from build123d import *


with BuildPart() as part:
    # Sketch1 → Revolve1 (revolve)
    with BuildSketch(Plane.XY, mode=Mode.PRIVATE) as revolve1_sk:
        Polygon((4.8, 24), (4.8, 22), (8.8, 22), (8.8, 20), (4.8, 20.000000056), (4.8, 18), (4.8, 16), (8.8, 16), (8.8, 14), (4.8, 14), (4.8, 11), (4.8, 10), (8.8, 10), (8.8, 8), (4.8, 8), (4.8, 5), (4.8, 4), (8.8, 4), (8.8, 2), (4.8, 2), (4.8, -1), (4.8, -2), (8.8, -2), (8.8, -4), (4.8, -4), (4.8, -7), (4.8, -8), (8.8, -8), (8.8, -10), (4.8, -10), (4.8, -13), (4.8, -14), (8.8, -14), (8.8, -16), (4.8, -16), (4.8, -19), (4.8, -20), (8.8, -20), (8.8, -22), (4.8, -22), (4.8, -24), (4.8, -27), (0, -27), (0, 27), (4.8, 27), align=None)
    revolve(revolve1_sk.sketch.rotate(Axis((0, 27, 0), (0, -1, 0)), 180), axis=Axis((0, 27, 0), (0, -1, 0)))


solid = part.part
The model under review builds one solid part; all positions refer to its coordinate system, in mm. A direction names the side the tool comes from. Give positions to 0.01 mm unless a question says otherwise; leave off trailing zeros. Order: outer loops, then holes, each group sorted by start corner. A loop starts at its lowest first (then second) coordinate and runs counter-clockwise, first axis right, second up. Notation, with made-up numbers: M 82.5,8.5 L 133.5,8.5 A10 cw 133.5,14.5 Z; hole C 56,2 d4. An arc over 180 degrees is marked long. One line per question, with ' | ' between items. Start each with the question number.
1) Clearance check with a flat-ended pin moving along its axis: P1, Ø5, axis at y = 17, z = 6, coming from the -X side. State where the tip first meets the part, or that it passes through.
2) Consider section C-C, the plane y = 21.5. Give the boundary of the cut face in (x, z), then the cut area to 3 significant figures.
3) Mouldability with a two-part tool opening along Y and no side actions: class faces 6 (the face through (1.146, 20.986, -8.725)), 7 (the face through (4, 16, 4)), 8 (the face through (0, 27, 0)) as pulls with the +Y half, pulls with the -Y half, needs draft (parallel to the pull), parting line crosses it, or undercut.
4) For faces 1 (the face through (4, -14, 4)), 2 (the face through (-4, -22, 4)), 3 (the face through (1.146, 2.986, -8.725)), 4 (the face through (0, -27, 0)), 5 (the face through (-2.58, 24.54, -4.05)), list the 3-axis set-ups (+Z, -Z, +X, -X, +Y, -Y) from which the entire face can be reached by the end or side of a thin tool; tool diameter is ignored.
5) Consider section D-D, the plane y = 5.5. Give the boundary of the cut face in (x, z), then the cut area to 3 significant figures.
6) Wall thickness on L1, parallel to X at y = -5.5, z = 0.25; L2, parallel to X at y = -23.5, z = -4.25; L3, parallel to Z at x = 2.75, y = -7: over which ranges is each line inside the solid? List them lowest first. Write a range as from..to.
7) Consider section A-A, the plane z = -6.5. State how many separate pieces and enclosed holes the cut face has, then the cut area to 3 significant figures.
Found:
1) P1: stops at x = -7.98
2) outline: C 0,0 d17.6 | area: 243 mm²
3) face 6: needs draft | face 7: undercut | face 8: pulls with the +Y half
4) face 1: none | face 2: -Y | face 3: +Y, -Y | face 4: +Z, -Z, +X, -X, -Y | face 5: +Y
5) outline: C 0,0 d9.6 | area: 72.4 mm²
6) L1: x = -4.79..4.79 | L2: x = -2.23..2.23 | L3: z = -3.93..3.93
7) separate pieces: 8 | enclosed holes: 0 | area: 190 mm²
